```python
from build123d import *

# Parameters (mm, degrees)
SKETCH_R             = 11.2
SKETCH_R_2           = 3.15
SKETCH_R_3           = 1.65
PAD_DEPTH            = 5
PAD001_DEPTH         = 30
SKETCH002_R          = 3.15
POCKET_DEPTH         = 43.001
POCKET001_DEPTH      = 40.001
POCKET001_DEPTH_BACK = -40.001
FILLET_R             = 1
SKETCH004_R          = 0.5
POCKET002_DEPTH      = 5.001
POCKET002_DEPTH_BACK = -30.001


with BuildPart() as part:
    # Sketch → Pad (new body)
    with BuildSketch(Plane.XY):
        Polygon((-30, 40), (-30, -40), (5, -40), (5, -26.5), (43, -26.5), (43, 26.5), (5, 26.5), (5, 40), align=None)
        with Locations((22, 0)):
            Circle(SKETCH_R, mode=Mode.SUBTRACT)
        with Locations((-15, 30)):
            Circle(SKETCH_R_2, mode=Mode.SUBTRACT)
        with Locations((-15, -30)):
            Circle(SKETCH_R_2, mode=Mode.SUBTRACT)
        with Locations((6.5, -15.5)):
            Circle(SKETCH_R_3, mode=Mode.SUBTRACT)
        with Locations((37.5, -15.5)):
            Circle(SKETCH_R_3, mode=Mode.SUBTRACT)
        with Locations((37.5, 15.5)):
            Circle(SKETCH_R_3, mode=Mode.SUBTRACT)
        with Locations((6.5, 15.5)):
            Circle(SKETCH_R_3, mode=Mode.SUBTRACT)
    extrude(amount=-PAD_DEPTH)

    # Sketch001 → Pad001 (join)
    with BuildSketch(Plane.XY):
        Polygon((0, -40), (5, -40), (5, -26.5), (43, -26.5), (43, -21.5), (0, -21.5), align=None)
        Polygon((0, 21.5), (43, 21.5), (43, 26.5), (5, 26.5), (5, 40), (0, 40), align=None)
    extrude(amount=PAD001_DEPTH)

    # Sketch002 → Pocket (cut, through all)
    with BuildSketch(Plane.YZ):
        with Locations((-33.25, 15)):
            Circle(SKETCH002_R)
        with Locations((33.25, 15)):
            Circle(SKETCH002_R)
    extrude(amount=POCKET_DEPTH, mode=Mode.SUBTRACT)

    # Sketch003 → Pocket001 (cut, two sides)
    with BuildSketch(Plane.XZ) as pocket001_sk:
        Polygon((5, 30), (43, 30), (43, 0), align=None)
    extrude(amount=-POCKET001_DEPTH, mode=Mode.SUBTRACT)
    extrude(pocket001_sk.sketch, amount=-POCKET001_DEPTH_BACK, mode=Mode.SUBTRACT)

    # Fillet
    fillet_edges = [part.edges().sort_by_distance(p)[0] for p in [
        (5, -26.5, 12.5),
        (5, 26.5, 12.5),
        (43, 26.5, -2.5),
        (43, -26.5, -2.5),
        (0, -21.5, 15),
        (0, 21.5, 15),
        (5, -40, 12.5),
        (5, 40, 12.5),
        (-30, 40, -2.5),
        (-30, -40, -2.5),
    ]]
    fillet(fillet_edges, radius=FILLET_R)

    # Sketch004 (on Face2 of Fillet) → Pocket002 (cut, two sides)
    with BuildSketch(Plane.XY) as pocket002_sk:
        with Locations((-30, 0)):
            Circle(SKETCH004_R)
    extrude(amount=-POCKET002_DEPTH, mode=Mode.SUBTRACT)
    extrude(pocket002_sk.sketch, amount=-POCKET002_DEPTH_BACK, mode=Mode.SUBTRACT)


solid = part.part
```
The model under review builds one solid part; all positions refer to its coordinate system, in mm. A direction names the side the tool comes from. Round coordinates to 2 decimals unless told otherwise and drop trailing zeros. Loops run counter-clockwise (first coordinate to the right, second up) from the corner with the lowest first, then second, coordinate; pieces in that order, holes last.
Item 1: Take a section at D-D (x = 30.5). Write out the cut boundary in (y, z), then the cut area to 3 significant figures.
Determined:
outline: (-26.5, -5) - (-7.29, -5) - (-7.29, 0) - (-21.5, 0) - (-21.5, 9.87) - (-26.5, 9.87) - close; (7.29, -5) - (26.5, -5) - (26.5, 9.87) - (21.5, 9.87) - (21.5, 0) - (7.29, 0) - close
area: 291 mm2
Item 2: For faces 5 (the face through (5, 36, 13)), 6 (the face through (18, -21.5, 11)), 7 (the face through (-2, 1, 0)), list the 3-axis set-ups (+Z, -Z, +X, -X, +Y, -Y) from which the entire face can be reached by the end or side of a thin tool; tool diameter is ignored.
Determined:
face 5: +Z, -Z, +X, +Y
face 6: +Z, +X, -X
face 7: +Z, -X
Item 3: Take a section at C-C (z = 15). Write out the cut boundary in (x, y), then the cut area to 3 significant figures.
Determined:
outline: (0, -40) - (4, -40) arc R1 ccw to (5, -39) - (5, -36.4) - (0, -36.4) - close; (0, -30.1) - (5, -30.1) - (5, -27.5) arc R1 cw to (6, -26.5) - (24, -26.5) - (24, -21.5) - (1, -21.5) arc R1 ccw to (0, -22.5) - close; (0, 22.5) arc R1 ccw to (1, 21.5) - (24, 21.5) - (24, 26.5) - (6, 26.5) arc R1 cw to (5, 27.5) - (5, 30.1) - (0, 30.1) - close; (0, 36.4) - (5, 36.4) - (5, 39) arc R1 ccw to (4, 40) - (0, 40) - close
area: 312 mm2
Item 4: For line 1 (Y direction, x = 2, z = 15); line 2 (Y direction, x = 6.5, z = -1.1); line 3 (Y direction, x = -15, z = -3.3), list the stretches that pass through material, from the lowest coordinate up.
Determined:
line 1: y = -40 to -36.4, -30.1 to -21.5, 21.5 to 30.1, 36.4 to 40
line 2: y = -26.5 to -17.15, -13.85 to 13.85, 17.15 to 26.5
line 3: y = -40 to -33.15, -26.85 to 26.85, 33.15 to 40
Item 5: Clearance check with flat-ended pins moving along their axes: pin 1 Ø1.5 at (x, y) = (8, -8) entering from +Z; pin 2 Ø14 at (y, z) = (32.5, 15) entering from -X; pin 3 Ø6 at (y, z) = (30.5, 18) entering from +X. State where each tip first meets the part, or that it passes through.
Determined:
pin 1: stops at z = 0
pin 2: stops at x = 0
pin 3: stops at x = 5
Item 6: Take a section at B-B (x = -15). Write out the cut boundary in (y, z), then the cut area to 3 significant figures.
Determined:
outline: (-40, -5) - (-33.15, -5) - (-33.15, 0) - (-40, 0) - close; (-26.85, -5) - (26.85, -5) - (26.85, 0) - (-26.85, 0) - close; (33.15, -5) - (40, -5) - (40, 0) - (33.15, 0) - close
area: 337 mm2
Item 7: Mouldability with a two-part tool opening along Y and no side actions: class faces 1 (the face through (20, 26.5, 5)), 2 (the face through (17, 21.5, 11)), 3 (the face through (20, -26.5, 8)), 4 (the face through (-2, 1, -5)) as released by +Y, released by -Y, zero draft, split by the parting line, or undercut.
Determined:
face 1: released by +Y
face 2: undercut
face 3: released by -Y
face 4: zero draft
Item 8: Take a section at A-A (y = -15.5). Write out the cut boundary in (x, z), then the cut area to 3 significant figures.
Determined:
outline: (-30, -5) - (4.85, -5) - (4.85, 0) - (-30, 0) - close; (8.15, -5) - (35.85, -5) - (35.85, 0) - (8.15, 0) - close; (39.15, -5) - (43, -5) - (43, 0) - (39.15, 0) - close
area: 332 mm2
